Read the model definition and answer for the solid it produces. Units are mm, in the model's axes. A direction names the side the tool comes from. Coordinates: 2 decimals unless noted, no trailing zeros. Write each loop counter-clockwise with the first axis right and the second up, starting at its lowest first coordinate (ties: lowest second). Pieces come first, ordered by that corner, then holes. Notation, with made-up numbers: M -30,-38 L 16,-38 A18 ccw 16,-8 Z; hole C 11,27.5 d3. An arc over 180 degrees is marked long. Write item = value, one per line.
from build123d import *

# Parameters (mm, degrees)
SKETCH_1_W           = 60
SKETCH_1_H           = 60
EXTRUDE_1_DEPTH      = 7
SKETCH_3_W           = 25
SKETCH_3_H           = 25
EXTRUDE_2_DEPTH      = 51.5
EXTRUDE_START        = 12.5
EXTRUDE_3_DEPTH      = 25
CUT_EXTRUDE_START    = -64
SKETCH_7_W           = 25
SKETCH_7_H           = 6.25
CUT_EXTRUDE_3_DEPTH  = 25
EXTRUDE_4_DEPTH      = 25
EXTRUDE_4_DEPTH_BACK = 25
SKETCH_8_R           = 6.25


with BuildPart() as part:
    # 草图1 → 凸台-拉伸1 (new body)
    with BuildSketch(Plane(origin=(0, 0, 0), x_dir=(1, 0, 0), z_dir=(0, 1, 0))):
        Rectangle(SKETCH_1_W, SKETCH_1_H)
    extrude(amount=EXTRUDE_1_DEPTH)

    # 草图3 → 凸台-拉伸2 (add)
    with BuildSketch(Plane(origin=(0, 0, 0), x_dir=(1, 0, 0), z_dir=(0, 1, 0))):
        Rectangle(SKETCH_3_W, SKETCH_3_H)
    extrude(amount=-EXTRUDE_2_DEPTH)

    # 草图4 → 凸台-拉伸3 (add)
    with BuildSketch(Plane.XY.offset(EXTRUDE_START)):
        with BuildLine():
            Line((12.5, -51.5), (-12.5, -51.5))
            ThreePointArc((-12.5, -51.5), (0, -64), (12.5, -51.5))
        make_face()
    extrude(amount=-EXTRUDE_3_DEPTH)

    # 草图7 → 切除-拉伸3 (cut)
    with BuildSketch(Plane(origin=(0, 0, 0), x_dir=(1, 0, 0), z_dir=(0, 1, 0)).offset(CUT_EXTRUDE_START)):
        with Locations((0, 9.375)):
            Rectangle(SKETCH_7_W, SKETCH_7_H)
        with Locations((0, -9.375)):
            Rectangle(SKETCH_7_W, SKETCH_7_H)
    extrude(amount=CUT_EXTRUDE_3_DEPTH, mode=Mode.SUBTRACT)

    # 草图8 → 凸台-拉伸4 (add, two sides: drawn at the far end of the back side and taken through both)
    with BuildSketch(Plane.XY.offset(-EXTRUDE_4_DEPTH_BACK)):
        with Locations((0, -51.5)):
            Circle(SKETCH_8_R)
    extrude(amount=EXTRUDE_4_DEPTH + EXTRUDE_4_DEPTH_BACK)


solid = part.part
Item 1: Find section D-D (y = -9). Determine the outline of the cut face in (x, z).
Worked answers:
outline = M -12.5,-12.5 L 12.5,-12.5 L 12.5,12.5 L -12.5,12.5 Z
Item 2: Find section A-A (z = 7.5). Determine the outline of the cut face in (x, y).
Worked answers:
outline = M -30,0 L -12.5,0 L -12.5,-39 L 12.5,-39 L 12.5,0 L 30,0 L 30,7 L -30,7 Z; C 0,-51.5 d12.5
Item 3: Which of the six approach directions +Z, -Z, +X, -X, +Y, -Y give full straight-line access (tool end or side, diameter ignored) to faces 4 (the face through (0, -51, 25)), 5 (the face through (0, -39, 9)), 6 (the face through (0, -51, -25)), 7 (the face through (-6, -49, -6.25)), 8 (the face through (-12.5, -25, 0))?
Worked answers:
face_4 = +Z, +X, -X, -Y
face_5 = +Z, +X, -X
face_6 = -Z, +X, -X, -Y
face_7 = -Z
face_8 = +Z, -Z, -X, -Y
Item 4: Consider line 1 along Y through (x, z) = (-20.5, -20.5); line 2 along Z through (x, y) = (-7, -36); line 3 along Z through (x, y) = (-8, -39.5). Determine where each line is inside the solid, lowest interval first. Write a range as from..to.
Worked answers:
line_1 = 0..7
line_2 = -12.5..12.5
line_3 = -6.25..6.25
Item 5: For a pull along Y with two mould halves and no side action, classify faces 1 (the face through (-6, -49, 6.25)), 2 (the face through (0, 3, -30)), 3 (the face through (0, 7, 0)) as released by +Y, released by -Y, zero draft, split by the parting line, or undercut.
Worked answers:
face_1 = undercut
face_2 = zero draft
face_3 = released by +Y
Item 6: Find section B-B (x = 11). Determine the outline of the cut face in (y, z).
Worked answers:
outline = M -57.44,-6.25 L -39,-6.25 L -39,-12.5 L 0,-12.5 L 0,-30 L 7,-30 L 7,30 L 0,30 L 0,12.5 L -39,12.5 L -39,6.25 L -57.44,6.25 Z
Item 7: Flat-ended cylindrical pins translate along their axes: pin 1 (5 mm diameter, centred on x = -3, z = 8.5, fed in from -Y); pin 2 (6 mm diameter, centred on x = 2, y = -54, fed in from +Z); pin 3 (20 mm diameter, centred on y = -13.5, z = 5, fed in from -X); pin 4 (4 mm diameter, centred on x = 16, y = -10.5, fed in from -Z). Find the tip coordinate at first contact, or state that the pin passes through.
Worked answers:
pin_1 = -63.85
pin_2 = 25
pin_3 = -12.5
pin_4 = through
Item 8: Find section C-C (z = -5). Determine the outline of the cut face in (x, y), and give its area (3 significant figures).
Worked answers:
outline = M -30,0 L -12.5,0 L -12.5,-51.5 A12.5 ccw 12.5,-51.5 L 12.5,0 L 30,0 L 30,7 L -30,7 Z
area = 1,950 mm²
